```python
from build123d import *

# Parameters (mm, degrees)
F0_W      = 177.8
F0_H      = 19.05
F1_DEPTH  = 6.35
F2_W      = 38.1
F2_H      = 31.75
F2_W_2    = 25.4
F2_H_2    = 19.05
F3_DEPTH  = 31.75
F4_W      = 25.4
F4_H      = 19.05
F5_DEPTH  = 127
F6_W      = 12.7
F6_H      = 5.08
F7_DEPTH  = 31.75
F9_DEPTH  = 12.7
F10_W     = 63.5
F10_H     = 12.7
F11_DEPTH = 31.751


with BuildPart() as f1:
    # F0 (on Front) → F1 (new body, symmetric)
    with BuildSketch(Plane.XZ):
        Rectangle(F0_W, F0_H)
    extrude(amount=F1_DEPTH, both=True)

    # F2 (on face) → F3 (join)
    with BuildSketch(Plane.XY.offset(9.525)):
        with Locations((-76.2, 0)):
            Rectangle(F2_W, F2_H)
        with Locations((-76.2, 0)):
            Rectangle(F2_W_2, F2_H_2, mode=Mode.SUBTRACT)
    extrude(amount=-F3_DEPTH)

    # F4 (on face) → F5 (cut)
    with BuildSketch(Plane.XY.offset(9.525)):
        with Locations((-76.2, 0)):
            Rectangle(F4_W, F4_H)
    extrude(amount=-F5_DEPTH, mode=Mode.SUBTRACT)

    # F6 (on face) → F7 (join)
    with BuildSketch(Plane.XY.offset(9.525)):
        with Locations((-76.2, 6.985)):
            Rectangle(F6_W, F6_H)
    extrude(amount=-F7_DEPTH)

    # F8 (on face) → F9 (join)
    with BuildSketch(Plane.XZ.offset(6.35)):
        Polygon((-57.15, -22.225), (-31.829141, -9.525), (-57.15, -9.525), align=None)
    extrude(amount=-F9_DEPTH)

    # F10 (on face) → F11 (cut, through all)
    with BuildSketch(Plane.XY.offset(9.525)):
        with Locations((57.15, 0)):
            Rectangle(F10_W, F10_H)
    extrude(amount=-F11_DEPTH, mode=Mode.SUBTRACT)


solid = f1.part
```
Work out the finished part from the listing and answer in its coordinate system (mm). A direction names the side the tool comes from. Round coordinates to 2 decimals unless told otherwise and drop trailing zeros. Loops run counter-clockwise (first coordinate to the right, second up) from the corner with the lowest first, then second, coordinate; pieces in that order, holes last. Notation, with made-up numbers: (42, 85.25) -> (80, 85.25) arc R15 cw to (80, 99.25) -> close; hole circle Ø10 at (76.5, -18.5). An arc over 180 degrees is marked (long way). Write each question's results on one line, items separated by ' | '. Start each with the question number.
1. Section B-B (x = -67.5) is taken. Determine the outline of the cut face in (y, z) (3 decimals), plus the area to 3 significant figures.
2. Section A-A (y = -4.5) is taken. Determine the outline of the cut face in (x, z) (3 decimals).
3. Given pin 1 Ø10 at (x, y) = (7, -2.5) entering from -Z (3 decimals); pin 2 Ø1.5 at (y, z) = (-9, -4) entering from +X; pin 3 Ø8 at (y, z) = (11, -17) entering from +X, each flat-ended and moving along its own axis, determine where each tip first touches the part or whether it passes through.
4. Section D-D (y = 8) is taken. Determine the outline of the cut face in (x, z) (3 decimals).
5. Find the intervals of material crossed by probe 1 along X at (y, z) = (8, -5); probe 2 along X at (y, z) = (1, 7.5); probe 3 along Y at (x, z) = (-70, -7) (3 decimals), in increasing order. Write a range as from..to.
6. Section C-C (z = -5) is taken. Determine the outline of the cut face in (x, y) (3 decimals), plus the area to 3 significant figures.
7. A tool of negligible diameter and unlimited length cuts with its end or side. For faces 1 (the face through (-16, -6.35, 1)), 2 (the face through (-57.15, 11, -6)), 3 (the face through (-76, 4.445, -6)), from which of +Z, -Z, +X, -X, +Y, -Y can it reach the whole face along a straight path? Write none if from no direction.
Evaluation:
1) outline: (-15.875, -22.225) -> (-9.525, -22.225) -> (-9.525, 9.525) -> (-15.875, 9.525) -> close; (9.525, -22.225) -> (15.875, -22.225) -> (15.875, 9.525) -> (9.525, 9.525) -> close | area: 403 mm2
2) outline: (-95.25, -22.225) -> (-88.9, -22.225) -> (-88.9, 9.525) -> (-95.25, 9.525) -> close; (-63.5, -22.225) -> (-57.15, -22.225) -> (-31.829, -9.525) -> (25.4, -9.525) -> (25.4, 9.525) -> (-63.5, 9.525) -> close
3) pin 1: stops at z = -9.525 | pin 2: stops at x = -57.15 | pin 3: stops at x = -57.15
4) outline: (-95.25, -22.225) -> (-88.9, -22.225) -> (-88.9, 9.525) -> (-95.25, 9.525) -> close; (-82.55, -22.225) -> (-69.85, -22.225) -> (-69.85, 9.525) -> (-82.55, 9.525) -> close; (-63.5, -22.225) -> (-57.15, -22.225) -> (-57.15, 9.525) -> (-63.5, 9.525) -> close
5) probe 1: x = -95.25..-88.9, -82.55..-69.85, -63.5..-57.15 | probe 2: x = -95.25..-88.9, -63.5..25.4 | probe 3: y = -15.875..-9.525, 4.445..15.875
6) outline: (-95.25, -15.875) -> (-57.15, -15.875) -> (-57.15, -6.35) -> (25.4, -6.35) -> (25.4, 6.35) -> (-57.15, 6.35) -> (-57.15, 15.875) -> (-95.25, 15.875) -> close; hole (-88.9, -9.525) -> (-63.5, -9.525) -> (-63.5, 9.525) -> (-69.85, 9.525) -> (-69.85, 4.445) -> (-82.55, 4.445) -> (-82.55, 9.525) -> (-88.9, 9.525) -> close | area: 1,840 mm2
7) face 1: +Z, -Z, +X, -Y | face 2: +Z, -Z, +X, +Y | face 3: +Z, -Z
